Geometry check sheet. Reference: drawing and pictorial views, mm from the part's lowest x, y, z. Round coordinates to 2 decimals unless told otherwise and drop trailing zeros. Loops run counter-clockwise (first coordinate to the right, second up) from the corner with the lowest first, then second, coordinate; pieces in that order, holes last. Notation, with made-up numbers: M 37.5,30.25 L 88.5,30.25 A30 ccw 88.5,66.25 Z; hole C 62.25,88 d2. An arc over 180 degrees is marked long. One line per question, with ' | ' between items. Start each with the question number.
(1) Go/stop test with flat-tipped pins: P1, Ø3, axis at x = 31, z = 3, coming from the +Y side; P2, Ø1.8, axis at y = 16, z = 0.5, coming from the +X side; P3, Ø1.3, axis at x = 17.5, z = 0.5, coming from the -Y side; P4, Ø0.5, axis at x = 19.5, z = 2, coming from the +Y side. Record where each tip stops, or that it passes through.
(2) Section check A-A (x = 44). Record the boundary of the cut face in (y, z).
(3) Section check B-B (y = 16). Record the boundary of the cut face in (x, z), and give its area (3 significant figures).
(4) Section check C-C (z = 4.4). Record the boundary of the cut face in (x, y).
(5) Thickness scan on probe 1 along Y at (x, z) = (55, 0.95); probe 2 along X at (y, z) = (14.5, 1.9); probe 3 along X at (y, z) = (8.25, 0.55). Record the ranges inside material, lowest first. Write a range as [from, to].
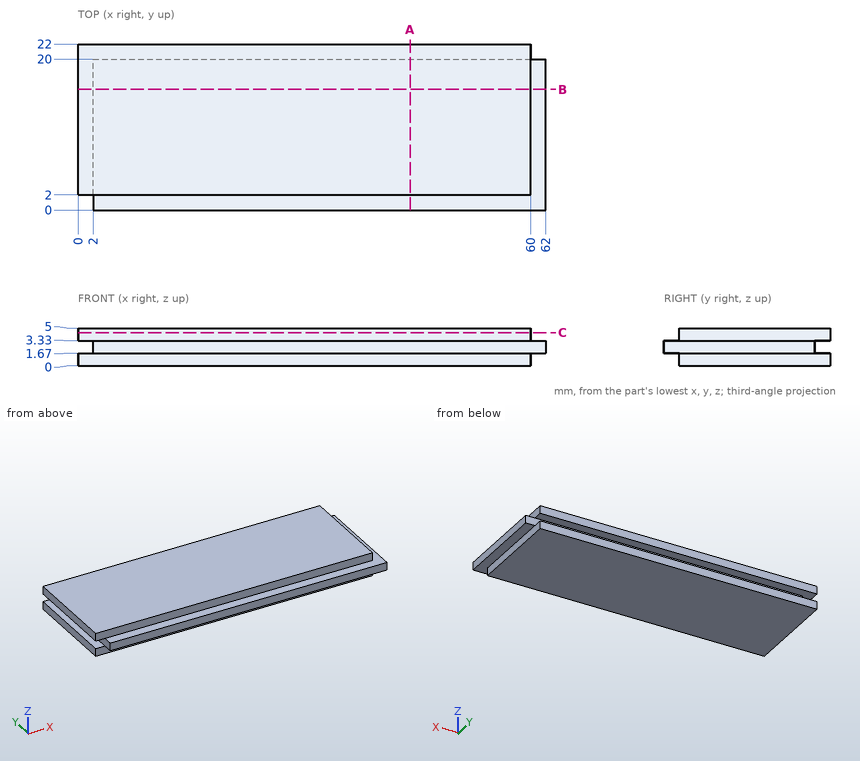
The answers:
1) P1: y = 22 | P2: x = 60 | P3: y = 2 | P4: y = 20
2) outline: M 0,1.67 L 2,1.67 L 2,0 L 22,0 L 22,1.67 L 20,1.67 L 20,3.33 L 22,3.33 L 22,5 L 2,5 L 2,3.33 L 0,3.33 Z
3) outline: M 0,0 L 60,0 L 60,1.67 L 62,1.67 L 62,3.33 L 60,3.33 L 60,5 L 0,5 L 0,3.33 L 2,3.33 L 2,1.67 L 0,1.67 Z | area: 300 mm²
4) outline: M 0,2 L 60,2 L 60,22 L 0,22 Z
5) probe 1: [2, 22] | probe 2: [2, 62] | probe 3: [0, 60]
